```python
from build123d import *

# Parameters (mm, degrees)
SKETCH_1_R               = 0.5
EXTRUDE_1_DEPTH          = 92
SHELL_1_T                = 1.5
EXTRUDE_2_OUTLINE_R      = 0.5
EXTRUDE_2_DEPTH          = 86
EXTRUDE_4_DEPTH          = 3
EXTRUDE_4_DEPTH_BACK     = 3
CUT_EXTRUDE_1_DEPTH      = 3
CUT_EXTRUDE_1_DEPTH_BACK = 3
CUT_EXTRUDE_2_DEPTH      = 10
CUT_EXTRUDE_2_DEPTH_BACK = 10
EXTRUDE_6_DEPTH          = 20
CUT_EXTRUDE_6_DEPTH      = 15
EXTRUDE_7_DEPTH          = 20
CUT_EXTRUDE_7_DEPTH      = 20


# Read off the part's stored shape, not the designer's step: 凸台-拉伸2
with BuildPart() as part:
    # 草图1 → 凸台-拉伸1 (new body)
    with BuildSketch(Plane(origin=(0, 0, 0), x_dir=(1, 0, 0), z_dir=(0, 1, 0))):
        with Locations(Location((0, 0, 0), (0, 0, 270))):
            Circle(SKETCH_1_R)
    extrude(amount=EXTRUDE_1_DEPTH)

    # 抽壳1
    shell_1_openings = [part.faces().sort_by_distance(p)[0] for p in [
        (0, 92, 0),
    ]]
    offset(amount=SHELL_1_T, openings=shell_1_openings, kind=Kind.INTERSECTION)

    # 凸台-拉伸2 outline → 凸台-拉伸2 (add)
    with BuildSketch(Plane(origin=(0, 0, 0), x_dir=(1, 0, 0), z_dir=(0, 1, 0))):
        Circle(EXTRUDE_2_OUTLINE_R)
    extrude(amount=EXTRUDE_2_DEPTH)

    # 草图5 → 凸台-拉伸4 (add, two sides: drawn at the far end of the back side and taken through both)
    with BuildSketch(Plane(origin=(0, 0, 0), x_dir=(0, 0, -1), z_dir=(1, 0, 0)).offset(-EXTRUDE_4_DEPTH_BACK)):
        Polygon((0, 38.5), (-15, 38.5), (0, -1.5), (15, 38.5), align=None)
    extrude(amount=EXTRUDE_4_DEPTH + EXTRUDE_4_DEPTH_BACK)

    # 草图6 → 切除-拉伸1 (cut, two sides: drawn at the far end of the back side and taken through both)
    with BuildSketch(Plane(origin=(0, 0, 0), x_dir=(0, 0, -1), z_dir=(1, 0, 0)).offset(-CUT_EXTRUDE_1_DEPTH_BACK)):
        Polygon((-2.867091748, -1.5), (0, -1.5), (-2.867091748, 6.145577994), align=None)
        Polygon((0, -1.5), (2.807839657, -1.5), (2.807839657, 5.987572419), align=None)
    extrude(amount=CUT_EXTRUDE_1_DEPTH + CUT_EXTRUDE_1_DEPTH_BACK, mode=Mode.SUBTRACT)

    # 草图8 → 切除-拉伸2 (cut, two sides: drawn at the far end of the back side and taken through both)
    with BuildSketch(Plane(origin=(0, 0, 0), x_dir=(0, 0, -1), z_dir=(1, 0, 0)).offset(-CUT_EXTRUDE_2_DEPTH_BACK)):
        Polygon((0, -1.5), (-1.055736005, 1.315296012), (1.055736005, 1.315296012), align=None)
    extrude(amount=CUT_EXTRUDE_2_DEPTH + CUT_EXTRUDE_2_DEPTH_BACK, mode=Mode.SUBTRACT)

    # 草图12 → 凸台-拉伸6 (add)
    with BuildSketch(Plane(origin=(3, 0, 0), x_dir=(0, 0, -1), z_dir=(1, 0, 0))):
        Polygon((1.055736005, 1.315296012), (-12.479805664, 38.5), (-15, 38.5), (-1.055736005, 1.315296012), align=None)
    extrude(amount=EXTRUDE_6_DEPTH)

    # 草图14 → 切除-拉伸6 (cut)
    with BuildSketch(Plane(origin=(0, 0.49322305, -1.354977403), x_dir=(-1, 0, 0), z_dir=(0, 0.3420517460280193, -0.939681117741111))):
        Polygon((-23, 40.446462351), (-3, 0.874842483), (-23, 0.874842483), align=None)
    extrude(amount=-CUT_EXTRUDE_6_DEPTH, mode=Mode.SUBTRACT)

    # 草图15 → 凸台-拉伸7 (add)
    with BuildSketch(Plane.ZY.offset(3)):
        Polygon((1.055736005, 1.315296012), (-12.756487539, 38.5), (-15, 38.5), (-1.055736005, 1.315296012), align=None)
    extrude(amount=EXTRUDE_7_DEPTH)

    # 草图16 → 切除-拉伸7 (cut)
    with BuildSketch(Plane(origin=(0, 0.504079298, 1.357061695), x_dir=(1, 0, 0), z_dir=(0, 0.3482034119031621, 0.9374190012683746))):
        Polygon((-3, 0.865372595), (-23, 40.532484034), (-23, 0.865372595), align=None)
    extrude(amount=-CUT_EXTRUDE_7_DEPTH, mode=Mode.SUBTRACT)


solid = part.part
```
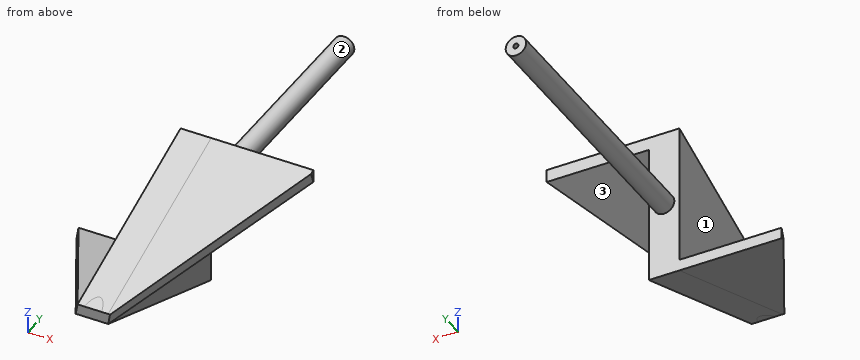
The listing builds one solid part. Answer for the finished solid, in the listing's coordinates (mm). Face numbers are marked on the shaded views. A direction names the side the tool comes from. Coordinates: 2 decimals unless noted, no trailing zeros. Loops run counter-clockwise (first coordinate to the right, second up) from the corner with the lowest first, then second, coordinate; pieces in that order, holes last. Notation, with made-up numbers: (8.5, 0) - (28.5, 0) arc R20 cw to (28.5, 24) - close; hole circle Ø4 at (11.25, -22.75). An arc over 180 degrees is marked (long way). Write item = value, one per line.
1) Section C-C (x = 19) is taken. Determine the outline of the cut face in (y, z), plus the area to 3 significant figures.
Responses:
outline = (30.28, 11.92) - (31.06, 9.77) - (38.5, 12.48) - (38.5, 15) - close
area = 19.4 mm^2
2) Section A-A (z = 7) is taken. Determine the outline of the cut face in (x, y), plus the area to 3 significant figures.
Responses:
outline = (-3, 17.17) - (11.92, 17.17) - (14.9, 23.45) - (3, 23.45) - (3, 38.5) - (-3, 38.5) - close
area = 193 mm^2
3) Find the intervals of material crossed by line 1 along X through (y, z) = (88.3, 0); line 2 along X through (y, z) = (43.5, -1.75); line 3 along Z through (x, y) = (-5.5, 35), in increasing order.
Responses:
line_1 = -2 to -0.5, 0.5 to 2
line_2 = -0.97 to 0.97
line_3 = -13.69 to -11.46
4) Section B-B (y = 50) is taken. Determine the outline of the cut face in (x, z), plus the area to 3 significant figures.
Responses:
outline = circle Ø4 at (0, 0)
area = 12.6 mm^2
5) Section D-D (z = -6) is taken. Determine the outline of the cut face in (x, y).
Responses:
outline = (-13.22, 20.31) - (-10.47, 14.5) - (3, 14.5) - (3, 38.5) - (-3, 38.5) - (-3, 20.31) - close
6) Which of the six approach directions +Z, -Z, +X, -X, +Y, -Y give full straight-line access (tool end or side, diameter ignored) to the marked faces 1, 2 and 3?
Responses:
face_1 = +Z, -X, +Y
face_2 = +Y
face_3 = -Z, +X, +Y
7) Each of these flat-tipped pins is pushed along its axis until it touches: P1, Ø8.5, axis at y = 22.5, z = 7.5, coming from the -X side; P2, Ø8, axis at x = -4.5, y = 47.5, coming from the +Z side; P3, Ø8, axis at y = 19.5, z = 1, coming from the +X side. Where does it stop, or does it pass through?
Responses:
P1 = -3
P2 = 1.94
P3 = 3
